For this review, take the finished solid that the model builds, in its own axes (mm). A direction names the side the tool comes from. Give positions to 0.01 mm unless a question says otherwise; leave off trailing zeros. Loops run counter-clockwise (first coordinate to the right, second up) from the corner with the lowest first, then second, coordinate; pieces in that order, holes last. Notation, with made-up numbers: (-39, 55.5) -> (-28, 55.5) arc R20 cw to (-28, 61.5) -> close; hole circle Ø6 at (8.5, -2.75). An arc over 180 degrees is marked (long way). One line per question, with ' | ' between items. Start each with the question number.
(1) Insertion check: P1, Ø15, axis at y = 69, z = -37.5, coming from the +X side; P2, Ø15, axis at y = 61.5, z = -37.5, coming from the -X side; P3, Ø1.2, axis at x = 735.5, z = 113.5, coming from the -Y side. Each pin has a flat end and moves straight along its axis. Give the tip position at first contact, or say it passes through.
(2) Consider section A-A (z = -40.5). Write out the cut boundary in (x, y), and give its area (4 significant figures).
(3) Consider section C-C (x = 213). Write out the cut boundary in (y, z).
(4) Draft analysis for pull direction X (two halves, no side actions). For faces 5 (the flat face through (533, 50, 95)), 6 (the flat face through (1027.5, 177, 91)), 7 (the flat face through (791.875, 108, 55)), 8 (the cylindrical face through (320.547, 65.21, -103.986)), state which applies: +X half, -X half, draft (parallel to the pull), parting line (faces both ways), or undercut.
(5) Consider section D-D (z = 51.5). Write out the cut boundary in (x, y) (3 decimals), and give its area (3 significant figures).
(6) Wall thickness on probe 1 along Y at (x, z) = (823, -35); probe 2 along Z at (x, y) = (340.5, 85.5); probe 3 along Z at (x, y) = (632.5, 175): over which ranges is each line inside the solid? List them lowest first.
(7) Tool access review of faces 1 (the flat face through (803, 80, -19)), 2 (the flat face through (811.875, 108, 55)), 3 (the flat face through (877.5, 65, -6)), 4 (the flat face through (326.25, 65, -6)): name each direction out of +Z, -Z, +X, -X, +Y, -Y from which nothing blocks a thin tool from reaching the whole face with its end or side.
(8) Consider section B-B (y = 149.5). Write out the cut boundary in (x, z) (3 decimals).
from build123d import *

# Parameters (mm, degrees)
EXTRUDE_1_DEPTH          = 1002.5
CUT_EXTRUDE_1_DEPTH      = 1058.062557278
CUT_EXTRUDE_1_DEPTH_BACK = 1058.062557278
SKETCH_2_W               = 400
SKETCH_2_H               = 185
CUT_EXTRUDE_2_DEPTH      = 1058.062557278
CUT_EXTRUDE_2_DEPTH_BACK = 1058.062557278
SKETCH_3_W               = 150
SKETCH_3_H               = 185
RIB_1_REACH              = 842.69
SKETCH_4_WALL_W          = 1799.999144386
SKETCH_4_WALL_H          = 20
RIB_2_REACH              = 842.69
SKETCH_5_WALL_W          = 1799.999144386
SKETCH_5_WALL_H          = 20
FILLET_2_R               = 20


with BuildPart() as part:
    # 草图1 → 凸台-拉伸1 (new body)
    with BuildSketch(Plane(origin=(1027.5, 0, 0), x_dir=(0, 0, -1), z_dir=(1, 0, 0))):
        Polygon((-105, 300), (-105, 180), (-110, 180), (-112.5, 185), (-115, 185), (-115, 165), (-112.5, 165), (-110, 170), (-105, 170), (-105, 50), (-75, 50), (110, 50), (110, 80), (-75, 80), (-75, 260), (-90, 300), align=None)
    extrude(amount=-EXTRUDE_1_DEPTH)

    # 草图2 → 切除-拉伸1 (cut, two sides: drawn at the far end of the back side and taken through both)
    with BuildSketch(Plane(origin=(0, 80, 0), x_dir=(1, 0, 0), z_dir=(0, 1, 0)).offset(-CUT_EXTRUDE_1_DEPTH_BACK)):
        with Locations((526.25, 17.5)):
            Rectangle(SKETCH_2_W, SKETCH_2_H)
    extrude(amount=CUT_EXTRUDE_1_DEPTH + CUT_EXTRUDE_1_DEPTH_BACK, mode=Mode.SUBTRACT)

    # 草图3 → 切除-拉伸2 (cut, two sides: drawn at the far end of the back side and taken through both)
    with BuildSketch(Plane(origin=(0, 80, 0), x_dir=(1, 0, 0), z_dir=(0, 1, 0)).offset(-CUT_EXTRUDE_2_DEPTH_BACK)):
        with Locations((100, 17.5)):
            Rectangle(SKETCH_3_W, SKETCH_3_H)
        with Locations((952.5, 17.5)):
            Rectangle(SKETCH_3_W, SKETCH_3_H)
    extrude(amount=CUT_EXTRUDE_2_DEPTH + CUT_EXTRUDE_2_DEPTH_BACK, mode=Mode.SUBTRACT)

    # 草图4 wall → 筋1 (add, up to next)
    with BuildSketch(Plane(origin=(801.875, 130, 45), x_dir=(0, 0.857492925713, 0.514495755428), z_dir=(0, -0.514495755428, 0.857492925713)), mode=Mode.PRIVATE) as rib_1_sk1:
        Rectangle(SKETCH_4_WALL_W, SKETCH_4_WALL_H)
    rib_1_tool1 = extrude(rib_1_sk1.sketch, amount=RIB_1_REACH, mode=Mode.PRIVATE) - part.part
    add(rib_1_tool1.solids().sort_by_distance((801.875, 130, 45))[0])

    # 草图5 wall → 筋2 (add, up to next)
    with BuildSketch(Plane(origin=(250.625, 130, 45), x_dir=(0, -0.857492925713, -0.514495755428), z_dir=(0, 0.514495755428, -0.857492925713)), mode=Mode.PRIVATE) as rib_2_sk1:
        Rectangle(SKETCH_5_WALL_W, SKETCH_5_WALL_H)
    rib_2_tool1 = extrude(rib_2_sk1.sketch, amount=-RIB_2_REACH, mode=Mode.PRIVATE) - part.part
    add(rib_2_tool1.solids().sort_by_distance((250.625, 130, 45))[0])

    # 圆角2
    fillet_2_edges = [part.edges().sort_by_distance(p)[0] for p in [
        (326.25, 65, -110),
        (726.25, 65, -110),
        (175, 65, -110),
        (877.5, 65, -110),
    ]]
    fillet(fillet_2_edges, radius=FILLET_2_R)


solid = part.part
A:
1) P1: stops at x = 877.5 | P2: stops at x = 175 | P3: stops at y = 165
2) outline: (175, 50) -> (326.25, 50) -> (326.25, 80) -> (175, 80) -> close; (726.25, 50) -> (877.5, 50) -> (877.5, 80) -> (726.25, 80) -> close | area: 9,075 mm^2
3) outline: (50, -110) -> (80, -110) -> (80, 75) -> (260, 75) -> (300, 90) -> (300, 105) -> (180, 105) -> (180, 110) -> (185, 112.5) -> (185, 115) -> (165, 115) -> (165, 112.5) -> (170, 110) -> (170, 105) -> (50, 105) -> close
4) face 5: draft | face 6: +X half | face 7: undercut | face 8: undercut
5) outline: (175, 50) -> (326.25, 50) -> (326.25, 80) -> (260.625, 80) -> (260.625, 140.833) -> (240.625, 140.833) -> (240.625, 80) -> (175, 80) -> close; (726.25, 50) -> (877.5, 50) -> (877.5, 80) -> (811.875, 80) -> (811.875, 140.833) -> (791.875, 140.833) -> (791.875, 80) -> (726.25, 80) -> close | area: 11,500 mm^2
6) probe 1: y = 50 to 80 | probe 2: z = 75 to 105 | probe 3: z = 75 to 115
7) face 1: -Z, +Y | face 2: -Z, +X, +Y | face 3: -Z, +X, +Y, -Y | face 4: -Z, +Y, -Y
8) outline: (25, 75) -> (240.625, 75) -> (240.625, 56.7) -> (260.625, 56.7) -> (260.625, 75) -> (791.875, 75) -> (791.875, 56.7) -> (811.875, 56.7) -> (811.875, 75) -> (1027.5, 75) -> (1027.5, 105) -> (25, 105) -> close
